Geometry check sheet. Reference: the model listing, model coordinates, mm. A direction names the side the tool comes from. Give positions to 0.01 mm unless a question says otherwise; leave off trailing zeros. Write each loop counter-clockwise with the first axis right and the second up, starting at its lowest first coordinate (ties: lowest second). Pieces come first, ordered by that corner, then holes. Notation, with made-up numbers: (21.5, -35) - (62.5, -35) arc R21 cw to (62.5, 3) - close; hole circle Ø5 at (57, 87.5). An arc over 180 degrees is marked (long way). Use a Markdown table: item, result.
```python
from build123d import *

# Parameters (mm, degrees)
BOSS_EXTRUDE1_DEPTH      = 4
BOSS_EXTRUDE1_DEPTH_BACK = 4
SKETCH1_R                = 22
SKETCH2_R                = 16
BOSS_EXTRUDE2_DEPTH      = 4
SKETCH3_R                = 18
BOSS_EXTRUDE3_DEPTH      = 12
BOSS_EXTRUDE4_START      = 3
SKETCH4_R                = 16
BOSS_EXTRUDE4_DEPTH      = 3
BOSS_EXTRUDE5_START      = 9
SKETCH5_R                = 18
BOSS_EXTRUDE5_DEPTH      = 9
CHAMFER1_SIZE            = 2
SKETCH6_R                = 12
CUT_EXTRUDE1_DEPTH       = 36


with BuildPart() as part:
    # Sketch1 → Boss-Extrude1 (new, two sides: drawn at the far end of the back side and taken through both)
    with BuildSketch(Plane(origin=(0, 0, 0), x_dir=(1, 0, 0), z_dir=(0, 1, 0)).offset(-BOSS_EXTRUDE1_DEPTH_BACK)):
        with Locations(Location((0, 0, 0), (0, 0, 270))):
            Circle(SKETCH1_R)
    extrude(amount=BOSS_EXTRUDE1_DEPTH + BOSS_EXTRUDE1_DEPTH_BACK)

    # Sketch2 → Boss-Extrude2 (add)
    with BuildSketch(Plane(origin=(0, 4, 0), x_dir=(1, 0, 0), z_dir=(0, 1, 0))):
        with Locations(Location((0, 0, 0), (0, 0, 270))):
            Circle(SKETCH2_R)
    extrude(amount=BOSS_EXTRUDE2_DEPTH)

    # Sketch3 → Boss-Extrude3 (add)
    with BuildSketch(Plane(origin=(0, 8, 0), x_dir=(1, 0, 0), z_dir=(0, 1, 0))):
        with Locations(Location((0, 0, 0), (0, 0, 270))):
            Circle(SKETCH3_R)
    extrude(amount=BOSS_EXTRUDE3_DEPTH)

    # Sketch4 → Boss-Extrude4 (add)
    with BuildSketch(Plane.XZ.offset(4).offset(BOSS_EXTRUDE4_START)):
        with Locations(Location((0, 0, 0), (0, 0, 90))):
            Circle(SKETCH4_R)
    extrude(amount=-BOSS_EXTRUDE4_DEPTH)

    # Sketch5 → Boss-Extrude5 (add)
    with BuildSketch(Plane.XZ.offset(7).offset(BOSS_EXTRUDE5_START)):
        with Locations(Location((0, 0, 0), (0, 0, 90))):
            Circle(SKETCH5_R)
    extrude(amount=-BOSS_EXTRUDE5_DEPTH)

    # Chamfer1
    chamfer1_edges = [part.edges().sort_by_distance(p)[0] for p in [
        (0, 20, -18),
    ]]
    chamfer(chamfer1_edges, length=CHAMFER1_SIZE)

    # Sketch6 → Cut-Extrude1 (cut)
    with BuildSketch(Plane(origin=(0, 20, 0), x_dir=(1, 0, 0), z_dir=(0, 1, 0))):
        with Locations(Location((0, 0, 0), (0, 0, 270))):
            Circle(SKETCH6_R)
    extrude(amount=-CUT_EXTRUDE1_DEPTH, mode=Mode.SUBTRACT)


solid = part.part
```
1) Mould release check, pull along Z, two halves, no side actions. Record for faces 1 (the cylindrical face through (3.604, 2.252, 11.446)), 2 (the flat face through (12, 20, 2)), 3 (the cylindrical face through (15.62, -5.52, -3.47)): pulls with the +Z half, pulls with the -Z half, needs draft (parallel to the pull), parting line crosses it, or undercut.
Working result:
| item | result |
|---|---|
| face 1 | undercut |
| face 2 | needs draft |
| face 3 | parting line crosses it |
2) Material ranges on L1, parallel to Y at x = 7.5, z = -16; L2, parallel to Y at x = 15, z = -9.5; L3, parallel to X at y = 4.5, z = 0, recorded low to high. Write a range as from..to.
Working result:
| item | result |
|---|---|
| L1 | y = -16..-7, -4..4, 8..18.33 |
| L2 | y = -16..-7, -4..4, 8..18.24 |
| L3 | x = -16..-12, 12..16 |
3) Set-up check for faces 4 (the cylindrical face through (-21.477, -0.056, -4.769)), 5 (the cylindrical face through (-5.407, -11.563, 17.169)), 6 (the flat face through (12, -16, 4)), 7 (the flat face through (11, -7, -12)), 8 (the cylindrical face through (5.407, 12.93, 17.169)): record each of +Z, -Z, +X, -X, +Y, -Y from which the full face is reachable in a straight line by a thin tool's end or side.
Working result:
| item | result |
|---|---|
| face 4 | +Y, -Y |
| face 5 | -Y |
| face 6 | +Z, -Z, +X, -X, -Y |
| face 7 | none |
| face 8 | +Y |
4) Section check C-C on y = 5.5. Record the boundary of the cut face in (x, z).
Working result:
| item | result |
|---|---|
| outline | circle Ø32 at (0, 0); hole circle Ø24 at (0, 0) |
5) Section check A-A on x = 0. Record the boundary of the cut face in (y, z).
Working result:
| item | result |
|---|---|
| outline | (-16, -18) - (-7, -18) - (-7, -16) - (-4, -16) - (-4, -22) - (4, -22) - (4, -16) - (8, -16) - (8, -18) - (18, -18) - (20, -16) - (20, -12) - (-16, -12) - close; (-16, 12) - (20, 12) - (20, 16) - (18, 18) - (8, 18) - (8, 16) - (4, 16) - (4, 22) - (-4, 22) - (-4, 16) - (-7, 16) - (-7, 18) - (-16, 18) - close |
6) Section check B-B on z = 0. Record the boundary of the cut face in (x, y), then the cut area to 3 significant figures.
Working result:
| item | result |
|---|---|
| outline | (-22, -4) - (-16, -4) - (-16, -7) - (-18, -7) - (-18, -16) - (-12, -16) - (-12, 20) - (-16, 20) - (-18, 18) - (-18, 8) - (-16, 8) - (-16, 4) - (-22, 4) - close; (12, -16) - (18, -16) - (18, -7) - (16, -7) - (16, -4) - (22, -4) - (22, 4) - (16, 4) - (16, 8) - (18, 8) - (18, 18) - (16, 20) - (12, 20) - close |
| area | 464 mm² |
7) Depth check by flat-ended pin: P1, Ø10, axis at x = -16.5, y = 14, coming from the +Z side; P2, Ø10, axis at y = 5, z = 4, coming from the -X side; P3, Ø10, axis at x = -2.5, y = -8.5, coming from the -Z side; P4, Ø18, axis at x = -7, z = -1.5, coming from the +Y side. Enter the tip coordinate at first touch or a pass-through.
Working result:
| item | result |
|---|---|
| P1 | stops at z = 13.85 |
| P2 | stops at x = -22 |
| P3 | stops at z = -22 |
| P4 | stops at y = 20 |
8) Section check D-D on y = 15. Record the boundary of the cut face in (x, z).
Working result:
| item | result |
|---|---|
| outline | circle Ø36 at (0, 0); hole circle Ø24 at (0, 0) |
